Part model, mm, in its own coordinate system. A direction names the side the tool comes from. Coordinates: 2 decimals unless noted, no trailing zeros. Order: outer loops, then holes, each group sorted by start corner. A loop starts at its lowest first (then second) coordinate and runs counter-clockwise, first axis right, second up.
from build123d import *

# Parameters (mm, degrees)
F2_DEPTH = 0.7
F3_DEPTH = 0.35
F5_D     = 4.2
F6_DEPTH = 1.25


with BuildPart() as f1:
    # F0 (on Front) → F1 (revolve)
    with BuildSketch(Plane.XZ):
        Polygon((-16, 84), (-16, 67), (16, 67), (16, 84), (16.35, 84), (16.35, 88), (-16.35, 88), (-16.35, 84), align=None)
    revolve(axis=Axis((-7.2666932824, 0, 0), (1, 0, 0)))

    # F2 (cut): a face of the model
    f2_faces = [f1.faces().sort_by_distance(p)[0] for p in [
        (16.35, 0, -86.4890158698),
    ]]
    extrude(f2_faces, amount=-F2_DEPTH, mode=Mode.SUBTRACT)

    # F3 (add): a face of the model
    f3_faces = [f1.faces().sort_by_distance(p)[0] for p in [
        (15.65, 0, -86.4890158698),
    ]]
    extrude(f3_faces, amount=F3_DEPTH)

    # F5 (through all)
    with Locations(Plane.YZ.offset(16)):
        with Locations((-67.9149415737, 38.9929093129), (0, 77.3538361923), (67.9149415737, 38.9929093129), (67.2629921577, -39.0070906871), (0, -78.5), (-67.2629921577, -39.0070906871)):
            Hole(F5_D / 2)

    # F6 (add): a face of the model
    f6_faces = [f1.faces().sort_by_distance(p)[0] for p in [
        (-16.35, 0, -85.5109841302),
    ]]
    extrude(f6_faces, amount=F6_DEPTH)


solid = f1.part
Q1. Mould opens along Y. For faces 3 (the face through (16, 65, 20)), 4 (the face through (-0.224, 1.666, -79.778)) say: pulls with the +Y half, pulls with the -Y half, needs draft (parallel to the pull), parting line crosses it, or undercut.
Results list:
face 3: needs draft
face 4: undercut
Q2. Cut at A-A on y = 0. Write the cut outline in (x, z).
Results list:
outline: (-17.6, -88) - (16, -88) - (16, -80.6) - (-16, -80.6) - (-16, -84) - (-17.6, -84) - close; (-17.6, 84) - (-16, 84) - (-16, 79.45) - (16, 79.45) - (16, 88) - (-17.6, 88) - close; (-16, -76.4) - (16, -76.4) - (16, -67) - (-16, -67) - close; (-16, 67) - (16, 67) - (16, 75.25) - (-16, 75.25) - close
Q3. Cut at D-D on x = -6. Write the cut outline in (y, z).
Results list:
outline: circle Ø176 at (0, 0); hole circle Ø4.2 at (-67.91, 38.99); hole circle Ø4.2 at (-67.26, -39.01); hole circle Ø134 at (0, 0); hole circle Ø4.2 at (0, -78.5); hole circle Ø4.2 at (0, 77.35); hole circle Ø4.2 at (67.26, -39.01); hole circle Ø4.2 at (67.91, 38.99)
Q4. Cut at C-C on y = 31. Write the cut outline in (x, z), and give its area (3 significant figures).
Results list:
outline: (-17.6, -82.36) - (16, -82.36) - (16, -59.4) - (-16, -59.4) - (-16, -78.07) - (-17.6, -78.07) - close; (-17.6, 78.07) - (-16, 78.07) - (-16, 59.4) - (16, 59.4) - (16, 82.36) - (-17.6, 82.36) - close
area: 1,480 mm2
Q5. Pin check, flat tips, straight feed: pin 1 Ø12 at (x, y) = (7.5, -65) entering from +Z; pin 2 Ø10 at (x, z) = (-9.5, -9.5) entering from -Y; pin 3 Ø5 at (y, z) = (67.91, 38.99) entering from +X; pin 4 Ø3 at (x, z) = (7.5, -53) entering from +Y. Stop position of each tip, or through.
Results list:
pin 1: stops at z = 65.29
pin 2: stops at y = -87.88
pin 3: stops at x = 16
pin 4: stops at y = 71.36
Q6. Wall check: line 1 along Z through (x, y) = (4, 0); line 2 along Y through (x, z) = (-16.85, 0); line 3 along Y through (x, z) = (-1, 0). Give the ranges that are in metal, low to high.
Results list:
line 1: z = -88 to -80.6, -76.4 to -67, 67 to 75.25, 79.45 to 88
line 2: y = -88 to -84, 84 to 88
line 3: y = -88 to -67, 67 to 88
Q7. Cut at B-B on z = 0. Write the cut outline in (x, y), and give its area (3 significant figures).
Results list:
outline: (-17.6, -88) - (16, -88) - (16, -67) - (-16, -67) - (-16, -84) - (-17.6, -84) - close; (-17.6, 84) - (-16, 84) - (-16, 67) - (16, 67) - (16, 88) - (-17.6, 88) - close
area: 1,360 mm2
Q8. Which spindle directions (+Z, -Z, +X, -X, +Y, -Y) get a long thin tool onto all of the face, cutting with end or side? Do faces 1 (the face through (-17.6, 32, 78)), 2 (the face through (-16, 24, -63)). Say none if no direction does.
Results list:
face 1: +Z, -Z, -X, +Y, -Y
face 2: -X
